from build123d import *

# Parameters (mm, degrees)
F0_W     = 130.8541893959
F0_H     = 56.7789375782
F1_DEPTH = 3
F3_DEPTH = 1.5
F4_R     = 14.2398683788
F5_DEPTH = 2
F7_D     = 7


# Not quite as in the source:
# - a feature names something its author has since deleted; it is built from what else it names


with BuildPart() as f1:
    # F0 (on Top) → F1 (new body)
    with BuildSketch(Plane.XY):
        Rectangle(F0_W, F0_H)
    extrude(amount=F1_DEPTH)

    # F2 (on face) → F3 (join)
    with BuildSketch(Plane.XY.offset(3)):
        with BuildLine():
            Line((57.2191747598, 28.3894687891), (53.5310418569, 28.3894687891))
            add(Edge.make_bspline(
                [(52.5161502643, 28.1952754595), (53.0025964919, 28.3138756826), (53.5310418569, 28.3894687891)],
                knots=[0, 0, 0, 0.3626225608, 0.3626225608, 0.3626225608], degree=2))
            add(Edge.make_bspline(
                [(50.0401853118, 27.2626364423), (51.1746831848, 27.8682130096), (52.5161502643, 28.1952754595)],
                knots=[0, 0, 0, 1, 1, 1], degree=2))
            add(Edge.make_bspline(
                [(47.1834992262, 25.1852788506), (48.9056874388, 26.657059875), (50.0401853118, 27.2626364423)],
                knots=[0, 0, 0, 1, 1, 1], degree=2))
            Line((47.1834992262, 25.1852788506), (49.8664333853, 22.0066406659))
            add(Edge.make_bspline(
                [(52.534036492, 23.7799323863), (51.2564487973, 23.1564695912), (49.8664333853, 22.0066406659)],
                knots=[0, 0, 0, 1, 1, 1], degree=2))
            add(Edge.make_bspline(
                [(55.1658671433, 24.4033951813), (53.8116241868, 24.4033951813), (52.534036492, 23.7799323863)],
                knots=[0, 0, 0, 1, 1, 1], degree=2))
            add(Edge.make_bspline(
                [(57.2355592089, 23.7160530015), (56.4587858905, 24.4033951813), (55.1658671433, 24.4033951813)],
                knots=[0, 0, 0, 1, 1, 1], degree=2))
            add(Edge.make_bspline(
                [(58.0123325273, 21.6233643575), (58.0123325273, 23.0287108217), (57.2355592089, 23.7160530015)],
                knots=[0, 0, 0, 1, 1, 1], degree=2))
            add(Edge.make_bspline(
                [(57.6597183236, 19.8040794801), (58.0123325273, 20.6830598141), (58.0123325273, 21.6233643575)],
                knots=[0, 0, 0, 1, 1, 1], degree=2))
            add(Edge.make_bspline(
                [(56.5098893983, 17.8953634641), (57.3071041198, 18.9250991461), (57.6597183236, 19.8040794801)],
                knots=[0, 0, 0, 1, 1, 1], degree=2))
            add(Edge.make_bspline(
                [(53.1063957793, 14.1980246753), (55.7126746767, 16.865627782), (56.5098893983, 17.8953634641)],
                knots=[0, 0, 0, 1, 1, 1], degree=2))
            Line((53.1063957793, 14.1980246753), (47.2448234356, 8.2751281222))
            Line((47.2448234356, 8.2751281222), (47.2448234356, 4.8409723986))
            Line((47.2448234356, 4.8409723986), (63.5672838243, 4.8409723986))
            Line((63.5672838243, 4.8409723986), (63.5672838243, 8.9956875821))
            Line((63.5672838243, 8.9956875821), (53.3925754229, 8.9956875821))
            Line((53.3925754229, 8.9956875821), (53.3925754229, 9.2154326656))
            Line((53.3925754229, 9.2154326656), (56.3974616811, 12.0414566465))
            add(Edge.make_bspline(
                [(60.58794932, 16.2753822671), (59.3972375885, 14.7908253657), (56.3974616811, 12.0414566465)],
                knots=[0, 0, 0, 1, 1, 1], degree=2))
            add(Edge.make_bspline(
                [(62.3459099881, 19.1729511588), (61.7786610516, 17.7599391684), (60.58794932, 16.2753822671)],
                knots=[0, 0, 0, 1, 1, 1], degree=2))
            add(Edge.make_bspline(
                [(62.9131589246, 22.2008339955), (62.9131589246, 20.5859631493), (62.3459099881, 19.1729511588)],
                knots=[0, 0, 0, 1, 1, 1], degree=2))
            add(Edge.make_bspline(
                [(61.9856302581, 25.4893447219), (62.9131589246, 24.0507809776), (62.9131589246, 22.2008339955)],
                knots=[0, 0, 0, 1, 1, 1], degree=2))
            add(Edge.make_bspline(
                [(59.3819065362, 27.7251231878), (61.0581015917, 26.9279084663), (61.9856302581, 25.4893447219)],
                knots=[0, 0, 0, 1, 1, 1], degree=2))
            add(Edge.make_bspline(
                [(57.2191747598, 28.3894687891), (58.3900152465, 28.1968763622), (59.3819065362, 27.7251231878)],
                knots=[0.4082482905, 0.4082482905, 0.4082482905, 1, 1, 1], degree=2))
        make_face()
        with BuildLine():
            Line((23.7372098514, 4.8409723986), (23.7372098514, 13.7994173145))
            Line((23.7372098514, 13.7994173145), (26.3690405026, 13.7994173145))
            Line((26.3690405026, 13.7994173145), (31.9444332027, 4.8409723986))
            Line((31.9444332027, 4.8409723986), (37.4380602903, 4.8409723986))
            add(Edge.make_bspline(
                [(30.5697488431, 15.0156808), (35.8436308472, 7.1406302493), (37.4380602903, 4.8409723986)],
                knots=[0, 0, 0, 1, 1, 1], degree=2))
            add(Edge.make_bspline(
                [(33.7816043078, 17.5299733833), (32.6496616103, 15.9253232387), (30.5697488431, 15.0156808)],
                knots=[0, 0, 0, 1, 1, 1], degree=2))
            add(Edge.make_bspline(
                [(34.9135470054, 21.194094892), (34.9135470054, 19.134623528), (33.7816043078, 17.5299733833)],
                knots=[0, 0, 0, 1, 1, 1], degree=2))
            add(Edge.make_bspline(
                [(32.6317753825, 26.4577561946), (34.9135470054, 24.7253472804), (34.9135470054, 21.194094892)],
                knots=[0, 0, 0, 1, 1, 1], degree=2))
            add(Edge.make_bspline(
                [(25.5871568334, 28.1901651087), (30.3500037596, 28.1901651087), (32.6317753825, 26.4577561946)],
                knots=[0, 0, 0, 1, 1, 1], degree=2))
            Line((25.5871568334, 28.1901651087), (18.7852799463, 28.1901651087))
            Line((18.7852799463, 28.1901651087), (18.7852799463, 4.8409723986))
            Line((18.7852799463, 4.8409723986), (23.7372098514, 4.8409723986))
        make_face()
        with BuildLine():
            Line((25.3316392945, 17.8263737285), (23.7372098514, 17.8263737285))
            Line((23.7372098514, 17.8263737285), (23.7372098514, 24.13254659))
            Line((23.7372098514, 24.13254659), (25.2396529804, 24.13254659))
            add(Edge.make_bspline(
                [(28.7734605442, 23.4298733579), (27.6312971451, 24.13254659), (25.2396529804, 24.13254659)],
                knots=[0, 0, 0, 1, 1, 1], degree=2))
            add(Edge.make_bspline(
                [(29.9156239434, 21.0663361225), (29.9156239434, 22.7272001258), (28.7734605442, 23.4298733579)],
                knots=[0, 0, 0, 1, 1, 1], degree=2))
            add(Edge.make_bspline(
                [(28.7990122981, 18.6082573977), (29.9156239434, 19.390141067), (29.9156239434, 21.0663361225)],
                knots=[0, 0, 0, 1, 1, 1], degree=2))
            add(Edge.make_bspline(
                [(25.3316392945, 17.8263737285), (27.6824006529, 17.8263737285), (28.7990122981, 18.6082573977)],
                knots=[0, 0, 0, 1, 1, 1], degree=2))
        make_face(mode=Mode.SUBTRACT)
        with BuildLine():
            add(Edge.make_bspline(
                [(13.9457777584, 16.5487860337), (13.9457777584, 10.7485378994), (11.0712054452, 7.6337790995)],
                knots=[0, 0, 0, 1, 1, 1], degree=2))
            add(Edge.make_bspline(
                [(11.0942020237, 25.4586826172), (13.9457777584, 22.3592548697), (13.9457777584, 16.5487860337)],
                knots=[0, 0, 0, 1, 1, 1], degree=2))
            add(Edge.make_bspline(
                [(5.2342333213, 28.3894687891), (8.9077868298, 27.8351356909), (11.0942020237, 25.4586826172)],
                knots=[0.2332606961, 0.2332606961, 0.2332606961, 1, 1, 1], degree=2))
            Line((5.2342333213, 28.3894687891), (0.4776699233, 28.3894687891))
            add(Edge.make_bspline(
                [(-5.4020102915, 25.4842343711), (-3.1948737915, 27.8381219683), (0.4776699233, 28.3894687891)],
                knots=[0, 0, 0, 0.7657718145, 0.7657718145, 0.7657718145], degree=2))
            add(Edge.make_bspline(
                [(-8.284248131, 16.5794481384), (-8.284248131, 22.4103583775), (-5.4020102915, 25.4842343711)],
                knots=[0, 0, 0, 1, 1, 1], degree=2))
            add(Edge.make_bspline(
                [(-5.4096758177, 7.6337790995), (-8.284248131, 10.7485378994), (-8.284248131, 16.5794481384)],
                knots=[0, 0, 0, 1, 1, 1], degree=2))
            add(Edge.make_bspline(
                [(2.8307648137, 4.5190202995), (-2.5351035044, 4.5190202995), (-5.4096758177, 7.6337790995)],
                knots=[0, 0, 0, 1, 1, 1], degree=2))
            add(Edge.make_bspline(
                [(11.0712054452, 7.6337790995), (8.1966331319, 4.5190202995), (2.8307648137, 4.5190202995)],
                knots=[0, 0, 0, 1, 1, 1], degree=2))
        make_face()
        with BuildLine():
            add(Edge.make_bspline(
                [(-3.0921317393, 16.5487860337), (-3.0921317393, 12.6342573369), (-1.607574838, 10.65399641)],
                knots=[0, 0, 0, 1, 1, 1], degree=2))
            add(Edge.make_bspline(
                [(-1.5922437857, 22.4461308329), (-3.0921317393, 20.4582043798), (-3.0921317393, 16.5487860337)],
                knots=[0, 0, 0, 1, 1, 1], degree=2))
            add(Edge.make_bspline(
                [(2.8614269184, 24.434057286), (-0.092355832, 24.434057286), (-1.5922437857, 22.4461308329)],
                knots=[0, 0, 0, 1, 1, 1], degree=2))
            add(Edge.make_bspline(
                [(8.7536613668, 16.5487860337), (8.7536613668, 24.434057286), (2.8614269184, 24.434057286)],
                knots=[0, 0, 0, 1, 1, 1], degree=2))
            add(Edge.make_bspline(
                [(2.8307648137, 8.673735483), (8.7536613668, 8.673735483), (8.7536613668, 16.5487860337)],
                knots=[0, 0, 0, 1, 1, 1], degree=2))
            add(Edge.make_bspline(
                [(-1.607574838, 10.65399641), (-0.1230179366, 8.673735483), (2.8307648137, 8.673735483)],
                knots=[0, 0, 0, 1, 1, 1], degree=2))
        make_face(mode=Mode.SUBTRACT)
        Polygon((-22.1281883918, 4.8409723986), (-17.1762584868, 4.8409723986), (-17.1762584868, 24.0712223807), (-10.8394235206, 24.0712223807), (-10.8394235206, 28.1901651087), (-28.4701337088, 28.1901651087), (-28.4701337088, 24.0712223807), (-22.1281883918, 24.0712223807), align=None)
        Polygon((-44.664835328, 28.1901651087), (-44.664835328, 4.8409723986), (-30.2434254291, 4.8409723986), (-30.2434254291, 8.929253022), (-39.712905423, 8.929253022), (-39.712905423, 28.1901651087), align=None)
        Polygon((-62.9803325206, 4.8409723986), (-49.5349996205, 4.8409723986), (-49.5349996205, 8.929253022), (-58.0284026155, 8.929253022), (-58.0284026155, 14.9492462399), (-50.1226899601, 14.9492462399), (-50.1226899601, 19.0068647585), (-58.0284026155, 19.0068647585), (-58.0284026155, 24.13254659), (-49.5349996205, 24.13254659), (-49.5349996205, 28.1901651087), (-62.9803325206, 28.1901651087), align=None)
    extrude(amount=F3_DEPTH)

    # F4 (on face) → F5 (join)
    with BuildSketch(Plane.XY.offset(3)):
        with Locations((-65.427094698, 0)):
            Circle(F4_R)
    extrude(amount=-F5_DEPTH)

    # F7 (through all)
    with Locations(Plane.XY.offset(3)):
        with Locations((-69.8119476438, 0)):
            Hole(F7_D / 2)


solid = f1.part
Can you work these out from the model? Positions are in its coordinate system, mm. A direction names the side the tool comes from. Coordinates: 2 decimals unless noted, no trailing zeros. Write each loop counter-clockwise with the first axis right and the second up, starting at its lowest first coordinate (ties: lowest second). Pieces come first, ordered by that corner, then holes.
Q1. Imagine slicing it at C-C, the plane x = -14. List the corners of the cut face in (y, z) for me, plus the area to 3 significant figures.
Results found:
outline: (-28.39, 0) - (28.39, 0) - (28.39, 3) - (28.19, 3) - (28.19, 4.5) - (24.07, 4.5) - (24.07, 3) - (-28.39, 3) - close
area: 177 mm2
Q2. If we mould it in two halves opening along Y, with no side actions, what happens to faces 1 (the face through (3, 17, 3)), 2 (the face through (-1, 28.389, 2)), 3 (the face through (-74, 0, 1))? For each: +Y half, -Y half, draft (parallel to the pull), parting line (faces both ways), or undercut.
Results found:
face 1: undercut
face 2: +Y half
face 3: draft
Q3. Imagine slicing it at B-B, the plane x = -68.5. List the corners of the cut face in (y, z) for me.
Results found:
outline: (-13.9, 1) - (-3.24, 1) - (-3.24, 3) - (-13.9, 3) - close; (3.24, 1) - (13.9, 1) - (13.9, 3) - (3.24, 3) - close
Q4. For P1, Ø1.6, axis at x = 24.5, z = 4, coming from the +Y side; P2, Ø1.6, axis at y = 6.5, z = 4, coming from the +X side; P3, Ø1.6, axis at x = -24.5, z = 4, coming from the -Y side, each with a flat end and sliding along its axis, tell me the tip position at first contact or that it passes through.
Results found:
P1: stops at y = 28.19
P2: stops at x = 63.57
P3: stops at y = 24.07
Q5. Which directions (+Z, -Z, +X, -X, +Y, -Y) give clear straight access to the entire face, cutting with the end or side of a thin tool? Please do faces 4 (the face through (-65.427, -0.4, 0.8)), 5 (the face through (48.506, 23.618, 3.74)), 6 (the face through (29.12, 9.38, 3.74)), 7 (the face through (55, 14, 4.5)), 8 (the face through (-66.315, 0.154, 1.986)).
Results found:
face 4: -Z, -X
face 5: +Z
face 6: +Z, -Y
face 7: +Z, +X, -X, +Y, -Y
face 8: +Z, -Z
Q6. Imagine slicing it at A-A, the plane y = 0. List the corners of the cut face in (x, z) for me, plus the area to 3 significant figures.
Results found:
outline: (-79.67, 1) - (-73.31, 1) - (-73.31, 3) - (-79.67, 3) - close; (-66.31, 1) - (-65.43, 1) - (-65.43, 0) - (65.43, 0) - (65.43, 3) - (-66.31, 3) - close
area: 407 mm2
Q7. Imagine slicing it at D-D, the plane y = -25. List the corners of the cut face in (x, z) for me, plus the area to 3 significant figures.
Results found:
outline: (-65.43, 0) - (65.43, 0) - (65.43, 3) - (-65.43, 3) - close
area: 393 mm2
Q8. Please list where these lines run through material, in increasing order: L1, parallel to Y at x = -55.5, z = 4.35; L2, parallel to X at y = 5, z = 0.7; L3, parallel to Z at x = -51, y = -4.5.
Results found:
L1: y = 4.84 to 8.93, 14.95 to 19.01, 24.13 to 28.19
L2: x = -65.43 to 65.43
L3: z = 0 to 3
